```python
from build123d import *

# Parameters (mm, degrees)
SKETCH2_R           = 22.5
BOSS_EXTRUDE1_DEPTH = 30
BOSS_EXTRUDE2_DEPTH = 20
CHAMFER1_START      = 18
CHAMFER1_OUTLINE_R  = 22.5
CHAMFER1_DEPTH      = 12
CHAMFER1_3_DEPTH    = 12
SKETCH8_R           = 3
CUT_EXTRUDE4_DEPTH  = 50
CUT_EXTRUDE5_DEPTH  = 10
SKETCH9_R           = 15
BOSS_EXTRUDE3_DEPTH = 2
DOME1_FACE_RADIUS   = 15
DOME1_HEIGHT        = 8
SKETCH13_R          = 1.5
CUT_EXTRUDE6_DEPTH  = 223.850286
SKETCH14_R          = 1
BOSS_EXTRUDE5_START = 16
SKETCH15_R          = 16
BOSS_EXTRUDE5_DEPTH = 16
SKETCH16_R          = 14
CUT_EXTRUDE7_DEPTH  = 20
SKETCH17_R          = 4
CUT_EXTRUDE8_DEPTH  = 2
CUT_EXTRUDE9_START  = -2
SKETCH18_R          = 4
CUT_EXTRUDE9_DEPTH  = 2
SKETCH19_R          = 3
CUT_EXTRUDE10_DEPTH = 221.132347


with BuildPart() as part:
    # Sketch2 → Boss-Extrude1 (new body)
    with BuildSketch(Plane(origin=(0, 0, 0), x_dir=(0, 0, -1), z_dir=(1, 0, 0))):
        Circle(SKETCH2_R)
    extrude(amount=BOSS_EXTRUDE1_DEPTH)

    # Sketch3 → Boss-Extrude2 (add)
    with BuildSketch(Plane(origin=(30, 0, 0), x_dir=(0, 0, -1), z_dir=(1, 0, 0))):
        with BuildLine():
            Line((-16, 0), (-16, 200))
            ThreePointArc((-16, 200), (0, 216), (16, 200))
            Line((16, 200), (16, 0))
            ThreePointArc((16, 0), (0, -16), (-16, 0))
        make_face()
    extrude(amount=BOSS_EXTRUDE2_DEPTH)

    # Chamfer1: read off the stored shape, not the designer's step
    # Chamfer1 outline → Chamfer1 (cut)
    with BuildSketch(Plane.YZ.offset(CHAMFER1_START)):
        Circle(CHAMFER1_OUTLINE_R)
    extrude(amount=CHAMFER1_DEPTH, mode=Mode.SUBTRACT)

    # Chamfer1 2 outline → Chamfer1 2 (revolve)
    with BuildSketch(Plane.YX):
        Polygon((0, 18), (22.5, 18), (15.999995, 24.500005), (0, 24.500005), align=None)
    revolve(axis=Axis((0, 0, 0), (1, 0, 0)))

    # Chamfer1 3 outline → Chamfer1 3 (add)
    with BuildSketch(Plane.YZ.offset(CHAMFER1_START)):
        with BuildLine():
            ThreePointArc((15.819292, -16), (22.5, 0), (15.819292, 16))
            Line((15.819292, 16), (0, 16))
            ThreePointArc((0, 16), (-16, 0), (0, -16))
            Line((0, -16), (15.819292, -16))
        make_face()
    extrude(amount=CHAMFER1_3_DEPTH)

    # Sketch8 → Cut-Extrude4 (cut)
    with BuildSketch(Plane.ZY):
        Circle(SKETCH8_R)
    extrude(amount=-CUT_EXTRUDE4_DEPTH, mode=Mode.SUBTRACT)

    # Sketch12 → Cut-Extrude5 (cut)
    with BuildSketch(Plane(origin=(50, 0, 0), x_dir=(0, 0, -1), z_dir=(1, 0, 0))):
        with BuildLine():
            Line((-13, 200), (-13, 145))
            Line((-13, 145), (13, 145))
            Line((13, 145), (13, 200))
            ThreePointArc((13, 200), (0, 213), (-13, 200))
        make_face()
    extrude(amount=-CUT_EXTRUDE5_DEPTH, mode=Mode.SUBTRACT)

    # Sketch9 → Boss-Extrude3 (add)
    with BuildSketch(Plane(origin=(50, 0, 0), x_dir=(0, 0, -1), z_dir=(1, 0, 0))):
        Circle(SKETCH9_R)
    extrude(amount=BOSS_EXTRUDE3_DEPTH)

    # Dome1: an elliptical dome of height H over a round flat face of radius A is half a spheroid: the quarter ellipse of half axes A and H revolved about the face's axis
    with BuildSketch(Plane((52, 0, 0), x_dir=(0, 0, 1), z_dir=(0, 1, 0)), mode=Mode.PRIVATE) as dome1_quarter:
        Ellipse(DOME1_FACE_RADIUS, DOME1_HEIGHT)
        Rectangle(DOME1_FACE_RADIUS, DOME1_HEIGHT, align=(Align.MIN, Align.MIN), mode=Mode.INTERSECT)
    revolve(dome1_quarter.sketch, axis=Axis((52, 0, 0), (1, 0, 0)))

    # Sketch13 → Cut-Extrude6 (cut, through all)
    with BuildSketch(Plane(origin=(50, 0, 0), x_dir=(0, 0, -1), z_dir=(1, 0, 0))):
        with Locations(Location((0, 11.481393, 0), (0, 0, 180))):
            Circle(SKETCH13_R)
        with Locations(Location((8.118571, 8.118571, 0), (0, 0, 180))):
            Circle(SKETCH13_R)
        with Locations((11.481393, 0)):
            Circle(SKETCH13_R)
        with Locations(Location((8.118571, -8.118571, 0), (0, 0, 180))):
            Circle(SKETCH13_R)
        with Locations(Location((0, -11.481393, 0), (0, 0, 180))):
            Circle(SKETCH13_R)
        with Locations(Location((-8.118571, -8.118571, 0), (0, 0, 180))):
            Circle(SKETCH13_R)
        with Locations(Location((-11.481393, 0, 0), (0, 0, 180))):
            Circle(SKETCH13_R)
        with Locations(Location((-8.118571, 8.118571, 0), (0, 0, 180))):
            Circle(SKETCH13_R)
    extrude(amount=CUT_EXTRUDE6_DEPTH, mode=Mode.SUBTRACT)

    # Sketch14 → Cut-Revolve1 (revolve, cut)
    with BuildSketch(Plane.XY, mode=Mode.PRIVATE) as cut_revolve1_sk:
        with Locations((2.818776, 22.5)):
            Circle(SKETCH14_R)
    revolve(cut_revolve1_sk.sketch.rotate(Axis((0, 0, 0), (-1, 0, 0)), 90), axis=Axis((0, 0, 0), (-1, 0, 0)), mode=Mode.SUBTRACT)

    # Sketch15 → Boss-Extrude5 (add)
    with BuildSketch(Plane.ZY.offset(-30).offset(BOSS_EXTRUDE5_START)):
        with Locations((0, 200)):
            Circle(SKETCH15_R)
    extrude(amount=-BOSS_EXTRUDE5_DEPTH)

    # Sketch16 → Cut-Extrude7 (cut)
    with BuildSketch(Plane.ZY.offset(-14)):
        with Locations((0, 200)):
            Circle(SKETCH16_R)
    extrude(amount=-CUT_EXTRUDE7_DEPTH, mode=Mode.SUBTRACT)

    # Sketch17 → Cut-Extrude8 (cut)
    with BuildSketch(Plane.ZY.offset(-34)):
        with Locations((0, 200)):
            Circle(SKETCH17_R)
    extrude(amount=-CUT_EXTRUDE8_DEPTH, mode=Mode.SUBTRACT)

    # Sketch18 → Cut-Extrude9 (cut)
    with BuildSketch(Plane(origin=(40, 0, 0), x_dir=(0, 0, -1), z_dir=(1, 0, 0)).offset(CUT_EXTRUDE9_START)):
        with Locations(Location((0, 200, 0), (0, 0, 180))):
            Circle(SKETCH18_R)
    extrude(amount=CUT_EXTRUDE9_DEPTH, mode=Mode.SUBTRACT)

    # Sketch19 → Cut-Extrude10 (cut, through all)
    with BuildSketch(Plane.ZY.offset(-36)):
        with Locations((0, 200)):
            Circle(SKETCH19_R)
    extrude(amount=-CUT_EXTRUDE10_DEPTH, mode=Mode.SUBTRACT)


solid = part.part
```
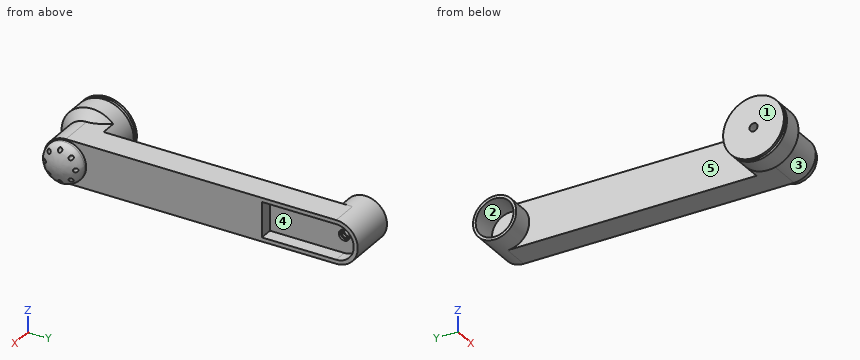
CAD build for the part. Positions are in the model's coordinates, mm. Face numbers are marked on the shaded views. A direction names the side the tool comes from. Coordinates: 2 decimals unless noted, no trailing zeros. Order: outer loops, then holes, each group sorted by start corner. A loop starts at its lowest first (then second) coordinate and runs counter-clockwise, first axis right, second up.
(1) Which spindle directions (+Z, -Z, +X, -X, +Y, -Y) get a long thin tool onto all of the face, cutting with end or side? Do the marked faces 1 and 2. Say none if no direction does.
Solution:
face 1: +Z, -Z, -X, +Y, -Y
face 2: -X
(2) Pin check, flat tips, straight feed: pin 1 Ø6 at (y, z) = (126, 5.5) entering from -X; pin 2 Ø2 at (y, z) = (49.5, -15) entering from +X; pin 3 Ø3.5 at (y, z) = (11.5, 0) entering from +X. Stop position of each tip, or through.
Solution:
pin 1: stops at x = 30
pin 2: stops at x = 50
pin 3: stops at x = 58.08
(3) Saw through at B-B, the plane y = 39.5. Write the cut outline in (x, z), and give its area (3 significant figures).
Solution:
outline: (30, -16) - (50, -16) - (50, 16) - (30, 16) - close
area: 640 mm2
(4) Drill centre lines: L1, parallel to Z at x = 39, y = 200; L2, parallel to Z at x = 42.5, y = 102.5; L3, parallel to Z at x = 36.75, y = 200. Where is each one in solid material? Low to high.
Solution:
L1: z = -16 to -4, 4 to 16
L2: z = -16 to 16
L3: z = -16 to -3, 3 to 16
(5) Mould opens along Z. For the marked faces 3, 4 and 5 say: released by +Z, released by -Z, zero draft, split by the parting line, or undercut.
Solution:
face 3: split by the parting line
face 4: undercut
face 5: zero draft
(6) Saw through at A-A, the plane x = 9. Write the cut outline in (y, z).
Solution:
outline: circle Ø45 at (0, 0); hole circle Ø6 at (0, 0)
